from build123d import *

# Parameters (mm, degrees)
CROQUIS2_R                   = 4
SALIENTE_EXTRUIR1_DEPTH      = 2
SALIENTE_EXTRUIR1_DEPTH_BACK = 2
CROQUIS2_3_R                 = 6
CROQUIS2_3_R_2               = 4
SALIENTE_EXTRUIR2_DEPTH      = 10
SALIENTE_EXTRUIR2_DEPTH_BACK = 10


with BuildPart() as part:
    # Croquis2 → Saliente-Extruir1 (new, two sides)
    with BuildSketch(Plane.XY) as saliente_extruir1_sk:
        with BuildLine():
            Line((7.5, 6), (7.5, -6))
            ThreePointArc((7.5, -6), (0, -13.5), (-7.5, -6))
            Line((-7.5, -6), (-7.5, 6))
            ThreePointArc((-7.5, 6), (0, 13.5), (7.5, 6))
        make_face()
        with Locations((0, -6)):
            Circle(CROQUIS2_R, mode=Mode.SUBTRACT)
        with Locations((0, 6)):
            Circle(CROQUIS2_R, mode=Mode.SUBTRACT)
    extrude(amount=SALIENTE_EXTRUIR1_DEPTH)
    extrude(saliente_extruir1_sk.sketch, amount=-SALIENTE_EXTRUIR1_DEPTH_BACK)

    # Croquis2_3 → Saliente-Extruir2 (add, two sides)
    with BuildSketch(Plane.XY) as saliente_extruir2_sk:
        with Locations((0, -6)):
            Circle(CROQUIS2_3_R)
        with Locations((0, -6)):
            Circle(CROQUIS2_3_R_2, mode=Mode.SUBTRACT)
    extrude(amount=SALIENTE_EXTRUIR2_DEPTH)
    extrude(saliente_extruir2_sk.sketch, amount=-SALIENTE_EXTRUIR2_DEPTH_BACK)


solid = part.part
Design review of the part built by this model. Coordinates are the model's own, in mm. A direction names the side the tool comes from. Round coordinates to 2 decimals unless told otherwise and drop trailing zeros. Write each loop counter-clockwise with the first axis right and the second up, starting at its lowest first coordinate (ties: lowest second). Pieces come first, ordered by that corner, then holes. Notation, with made-up numbers: (28.5, 62) -> (77.5, 62) arc R21 ccw to (77.5, 86) -> close; hole circle Ø1 at (-16, 32.25). An arc over 180 degrees is marked (long way). One line per question, with ' | ' between items.
(1) Machinability: for faces 1 (the cylindrical face through (-1.301, -11.857, 5.944)), 2 (the cylindrical face through (-1.301, -11.857, -5.944)), 3 (the flat face through (-7.5, 0, 0)), which of the approach directions +Z, -Z, +X, -X, +Y, -Y give a long, thin tool a straight path to every point of the face, cutting with its end or side? Answer none if there is none.
Result sheet:
face 1: +Z | face 2: -Z | face 3: +Z, -Z, -X, +Y, -Y
(2) Wall thickness on line 1 (Y direction, x = 0, z = 0.95); line 2 (Y direction, x = 0, z = -7); line 3 (Z direction, x = 5, y = 4.5): over which ranges is each line inside the solid? List them lowest first. Write a range as [from, to].
Result sheet:
line 1: [-13.5, -10], [-2, 2], [10, 13.5] | line 2: [-12, -10], [-2, 0] | line 3: [-2, 2]
(3) Insertion check: P1, Ø5, axis at x = 0, y = -2.5, coming from the -Z side; P2, Ø3, axis at x = 0, z = 5, coming from the -Y side; P3, Ø6.5, axis at x = 0, y = 6, coming from the +Z side; P4, Ø1.5, axis at x = 3, z = -6.5, coming from the +Y side. Each pin has a flat end and moves straight along its axis. Give the tip position at first contact, or say it passes through.
Result sheet:
P1: z = -10 | P2: y = -12 | P3: through | P4: y = -0.44
(4) Take a section at A-A, the plane x = 0. State the section outline as (y, z) points.
Result sheet:
outline: (-13.5, -2) -> (-12, -2) -> (-12, -10) -> (-10, -10) -> (-10, 10) -> (-12, 10) -> (-12, 2) -> (-13.5, 2) -> close; (-2, -10) -> (0, -10) -> (0, -2) -> (2, -2) -> (2, 2) -> (0, 2) -> (0, 10) -> (-2, 10) -> close; (10, -2) -> (13.5, -2) -> (13.5, 2) -> (10, 2) -> close
(5) Take a section at C-C, the plane z = -0.5. State the section outline as (x, y) points.
Result sheet:
outline: (-7.5, -6) arc R7.5 ccw to (7.5, -6) -> (7.5, 6) arc R7.5 ccw to (-7.5, 6) -> close; hole circle Ø8 at (0, -6); hole circle Ø8 at (0, 6)
(6) Take a section at D-D, the plane z = 7.75. State the section outline as (x, y) points.
Result sheet:
outline: circle Ø12 at (0, -6); hole circle Ø8 at (0, -6)
(7) Take a section at B-B, the plane y = 6.75. State the section outline as (x, z) points, and give its area (3 significant figures).
Result sheet:
outline: (-7.46, -2) -> (-3.93, -2) -> (-3.93, 2) -> (-7.46, 2) -> close; (3.93, -2) -> (7.46, -2) -> (7.46, 2) -> (3.93, 2) -> close | area: 28.3 mm2
